Input: part model. Units: mm. Frame: model coordinates. Face numbers are marked on the shaded views. A direction names the side the tool comes from. Coordinates: 2 decimals unless noted, no trailing zeros. Loops run counter-clockwise (first coordinate to the right, second up) from the corner with the lowest first, then second, coordinate; pieces in that order, holes last.
```python
from build123d import *

# Parameters (mm, degrees)
F1_DEPTH = 12.7
F2_DEPTH = 95.25


# Not quite as in the source:
# - a feature names something its author has since deleted; it is built from what else it names


with BuildPart() as f1:
    # F0 (on Front) → F1 (new body)
    with BuildSketch(Plane.XZ):
        Polygon((142.3687008922, 35.0424993012), (105.7069587986, 35.0424993011), (87.3760877519, 3.2924993012), (105.7069587986, -28.4575006988), (142.3687008922, -28.4575006988), (160.6995719389, 3.2924993012), align=None)
        Polygon((107.5400459033, -25.2825006989), (91.0422619612, 3.2924993011), (107.5400459033, 31.8674993011), (140.5356137875, 31.8674993012), (157.0333977296, 3.2924993012), (140.5356137875, -25.2825006988), align=None, mode=Mode.SUBTRACT)
        Polygon((105.7069587986, -28.4575006988), (87.3760877519, 3.2924993012), (50.7143456583, 3.2924993012), (32.3834746115, -28.4575006988), (50.7143456583, -60.2075006988), (87.3760877519, -60.2075006988), align=None)
        Polygon((52.547432763, -57.0325006988), (36.0496488209, -28.4575006988), (52.547432763, 0.1174993012), (85.5430006472, 0.1174993012), (102.0407845893, -28.4575006988), (85.5430006472, -57.0325006988), align=None, mode=Mode.SUBTRACT)
        Polygon((197.3613140325, 3.2924993012), (160.6995719389, 3.2924993012), (142.3687008922, -28.4575006988), (160.6995719389, -60.2075006988), (197.3613140325, -60.2075006988), (215.6921850793, -28.4575006988), align=None)
        Polygon((162.5326590436, -57.0325006988), (146.0348751015, -28.4575006988), (162.5326590436, 0.1174993012), (195.5282269278, 0.1174993012), (212.0260108699, -28.4575006988), (195.5282269278, -57.0325006988), align=None, mode=Mode.SUBTRACT)
        Polygon((142.3687008922, -28.4575006988), (105.7069587986, -28.4575006989), (87.3760877519, -60.2075006988), (105.7069587986, -91.9575006988), (142.3687008922, -91.9575006988), (160.6995719389, -60.2075006988), align=None)
        Polygon((107.5400459033, -88.7825006988), (91.0422619612, -60.2075006988), (107.5400459033, -31.6325006988), (140.5356137875, -31.6325006988), (157.0333977296, -60.2075006988), (140.5356137875, -88.7825006988), align=None, mode=Mode.SUBTRACT)
        Polygon((162.5326590436, 0.1174993012), (146.0348751015, -28.4575006988), (162.5326590436, -57.0325006988), (195.5282269278, -57.0325006988), (212.0260108699, -28.4575006988), (195.5282269278, 0.1174993012), align=None)
        Polygon((52.547432763, 0.1174993012), (36.0496488209, -28.4575006988), (52.547432763, -57.0325006988), (85.5430006472, -57.0325006988), (102.0407845893, -28.4575006988), (85.5430006472, 0.1174993012), align=None)
        Polygon((107.5400459033, 31.8674993011), (91.0422619612, 3.2924993011), (107.5400459033, -25.2825006989), (140.5356137875, -25.2825006988), (157.0333977296, 3.2924993012), (140.5356137875, 31.8674993012), align=None)
        Polygon((107.5400459033, -31.6325006988), (91.0422619612, -60.2075006988), (107.5400459033, -88.7825006988), (140.5356137875, -88.7825006988), (157.0333977296, -60.2075006988), (140.5356137875, -31.6325006988), align=None)
    extrude(amount=F1_DEPTH)

    # F0 (on Front) → F2 (join)
    with BuildSketch(Plane.XZ):
        Polygon((142.3687008922, 35.0424993012), (105.7069587986, 35.0424993011), (87.3760877519, 3.2924993012), (105.7069587986, -28.4575006988), (142.3687008922, -28.4575006988), (160.6995719389, 3.2924993012), align=None)
        Polygon((107.5400459033, -25.2825006989), (91.0422619612, 3.2924993011), (107.5400459033, 31.8674993011), (140.5356137875, 31.8674993012), (157.0333977296, 3.2924993012), (140.5356137875, -25.2825006988), align=None, mode=Mode.SUBTRACT)
        Polygon((197.3613140325, 3.2924993012), (160.6995719389, 3.2924993012), (142.3687008922, -28.4575006988), (160.6995719389, -60.2075006988), (197.3613140325, -60.2075006988), (215.6921850793, -28.4575006988), align=None)
        Polygon((162.5326590436, -57.0325006988), (146.0348751015, -28.4575006988), (162.5326590436, 0.1174993012), (195.5282269278, 0.1174993012), (212.0260108699, -28.4575006988), (195.5282269278, -57.0325006988), align=None, mode=Mode.SUBTRACT)
        Polygon((142.3687008922, -28.4575006988), (105.7069587986, -28.4575006989), (87.3760877519, -60.2075006988), (105.7069587986, -91.9575006988), (142.3687008922, -91.9575006988), (160.6995719389, -60.2075006988), align=None)
        Polygon((107.5400459033, -88.7825006988), (91.0422619612, -60.2075006988), (107.5400459033, -31.6325006988), (140.5356137875, -31.6325006988), (157.0333977296, -60.2075006988), (140.5356137875, -88.7825006988), align=None, mode=Mode.SUBTRACT)
        Polygon((105.7069587986, -28.4575006988), (87.3760877519, 3.2924993012), (50.7143456583, 3.2924993012), (32.3834746115, -28.4575006988), (50.7143456583, -60.2075006988), (87.3760877519, -60.2075006988), align=None)
        Polygon((52.547432763, -57.0325006988), (36.0496488209, -28.4575006988), (52.547432763, 0.1174993012), (85.5430006472, 0.1174993012), (102.0407845893, -28.4575006988), (85.5430006472, -57.0325006988), align=None, mode=Mode.SUBTRACT)
        Polygon((32.3834746115, -28.4575006988), (50.7143456583, 3.2924993012), (47.048171449, 3.2924993012), (28.7173004022, -28.4575006988), (48.8812585536, -63.3825006988), (85.5430006472, -63.3825006988), (103.873871694, -95.1325006988), (144.2017879969, -95.1325006988), (162.5326590436, -63.3825006988), (199.1944011372, -63.3825006988), (219.3583592886, -28.4575006988), (201.0274882418, 3.2924993011), (197.3613140325, 3.2924993012), (215.6921850793, -28.4575006988), (197.3613140325, -60.2075006988), (160.6995719389, -60.2075006988), (142.3687008922, -91.9575006988), (105.7069587986, -91.9575006988), (87.3760877519, -60.2075006988), (50.7143456583, -60.2075006988), align=None)
    extrude(amount=F2_DEPTH)


solid = f1.part
```
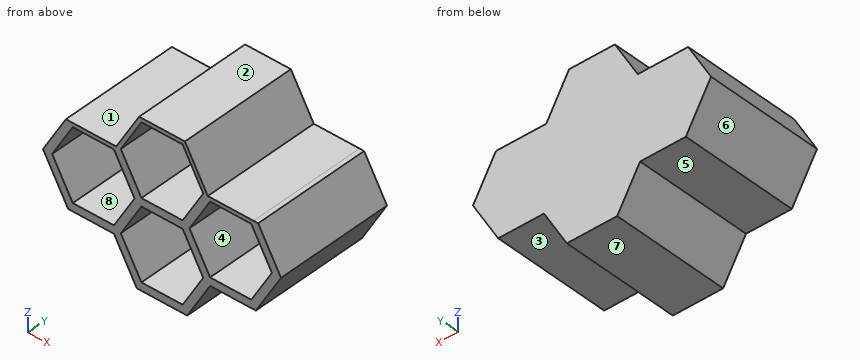
Item 1: Section query D-D (y = -20.5). Count the separate pieces of the cut face and the enclosed holes in it, then the cut area to 3 significant figures.
Result:
separate pieces: 1
enclosed holes: 4
area: 3,720 mm2
Item 2: Section query A-A (y = -8). Output: boundary loops of the cut face in (x, z), then the cut area to 3 significant figures.
Result:
outline: (28.72, -28.46) - (48.88, -63.38) - (85.54, -63.38) - (103.87, -95.13) - (144.2, -95.13) - (162.53, -63.38) - (199.19, -63.38) - (219.36, -28.46) - (201.03, 3.29) - (160.7, 3.29) - (142.37, 35.04) - (105.71, 35.04) - (87.38, 3.29) - (47.05, 3.29) - close
area: 15,000 mm2
Item 3: Line query: L1, parallel to Z at x = 138, y = -15; L2, parallel to Z at x = 53.5, y = -14.5; L3, parallel to X at y = -39, z = -50.5. Output: solid intervals per line, ascending.
Result:
L1: z = -95.13 to -88.78, -31.63 to -25.28, 31.87 to 35.04
L2: z = -63.38 to -57.03, 0.12 to 3.29
L3: x = 41.44 to 48.78, 89.31 to 96.65, 151.43 to 158.76, 199.3 to 206.63
Item 4: Section query C-C (z = -47.5). Output: boundary loops of the cut face in (x, y).
Result:
outline: (39.71, -95.25) - (47.04, -95.25) - (47.04, -12.7) - (91.05, -12.7) - (91.05, -95.25) - (98.38, -95.25) - (98.38, -12.7) - (149.7, -12.7) - (149.7, -95.25) - (157.03, -95.25) - (157.03, -12.7) - (201.03, -12.7) - (201.03, -95.25) - (208.36, -95.25) - (208.36, 0) - (39.71, 0) - close
Item 5: Contact query for flat-ended pins moving along their axis: P1, Ø5, axis at x = 76, z = -45.5, coming from the +Y side; P2, Ø18.5, axis at x = 65.5, y = -48, coming from the -Z side; P3, Ø4, axis at x = 93, y = -20, coming from the +Z side; P4, Ø8, axis at y = -85, z = 11, coming from the -X side. Output: stop coordinate, or through.
Result:
P1: stops at y = 0
P2: stops at z = -63.38
P3: stops at z = 16.5
P4: stops at x = 89.52
Item 6: Reachability of the marked faces 1, 2, 3, 4 and 5 from +Z, -Z, +X, -X, +Y, -Y: full face, straight path, thin tool, end or side. Return the list, or none.
Result:
face 1: +Z, -X, +Y, -Y
face 2: +Z, +X, -X, +Y, -Y
face 3: -Z, +X, +Y, -Y
face 4: -Y
face 5: -Z, -X, +Y, -Y
Item 7: Section query B-B (x = 68). Output: boundary loops of the cut face in (y, z).
Result:
outline: (-95.25, -63.38) - (0, -63.38) - (0, 3.29) - (-95.25, 3.29) - (-95.25, 0.12) - (-12.7, 0.12) - (-12.7, -57.03) - (-95.25, -57.03) - close
Item 8: Mould query, pull axis X, two halves, no side actions, for the marked faces 6, 7 and 8. Classes: +X half, -X half, draft (parallel to the pull), parting line (faces both ways), or undercut.
Result:
face 6: -X half
face 7: draft
face 8: undercut
